```python
from build123d import *

# Parameters (mm, degrees)
BOSS_EXTRUDE1_DEPTH = 11.5
SKETCH2_R           = 1
BOSS_EXTRUDE2_DEPTH = 1.5


with BuildPart() as part:
    # Sketch1 → Boss-Extrude1 (new body)
    with BuildSketch(Plane.XY):
        Polygon((7.5, 5.75), (-7.5, 5.75), (-7.5, -5.75), (-6, -5.75), (-6, 4.25), (6, 4.25), (6, -5.75), (7.5, -5.75), align=None)
    extrude(amount=-BOSS_EXTRUDE1_DEPTH)

    # Sketch2 → Boss-Extrude2 (add)
    with BuildSketch(Plane.XZ.offset(5.75)):
        with BuildLine():
            Line((-7.5, -10.75), (-7.5, -0.75))
            ThreePointArc((-7.5, -0.75), (-12.5, -5.75), (-7.5, -10.75))
        make_face()
        with Locations((-9.5, -4)):
            Circle(SKETCH2_R, mode=Mode.SUBTRACT)
        with BuildLine():
            Line((7.5, -0.75), (7.5, -10.75))
            ThreePointArc((7.5, -10.75), (12.5, -5.75), (7.5, -0.75))
        make_face()
        with Locations((9.5, -4)):
            Circle(SKETCH2_R, mode=Mode.SUBTRACT)
    extrude(amount=-BOSS_EXTRUDE2_DEPTH)


solid = part.part
```
Source: CAD feature listing. Evaluate the final solid. Frame: model axes, mm. A direction names the side the tool comes from. Give positions to 0.01 mm unless a question says otherwise; leave off trailing zeros. Loops run counter-clockwise (first coordinate to the right, second up) from the corner with the lowest first, then second, coordinate; pieces in that order, holes last. Notation, with made-up numbers: (-35, 17) - (-22, 17) arc R25 cw to (-22, 49) - close; hole circle Ø7 at (-3.5, 15). An arc over 180 degrees is marked (long way). Use CSV: the item, a comma, the result in double quotes. Start each with the question number.
1. Section C-C (z = -3.25). Output: boundary loops of the cut face in (x, y).
2. Reachability of faces 1 (the flat face through (9, -4.25, -6)), 2 (the flat face through (0, 5.75, -6)), 3 (the flat face through (6, -1, -6)), 4 (the flat face through (-9, -4.25, -6)) from +Z, -Z, +X, -X, +Y, -Y: full face, straight path, thin tool, end or side. Return the list, or none.
3. Section A-A (y = -2.5). Output: boundary loops of the cut face in (x, z).
4. Draft query along X for faces 5 (the flat face through (0, 4.25, -6)), 6 (the flat face through (8, -5.75, -6)), 7 (the cylindrical face through (8.763, -5.01, -3.324)), 8 (the cylindrical face through (12.5, -5.01, -5.86)). Return one class per face: +X half, -X half, draft (parallel to the pull), parting line (faces both ways), or undercut.
5. Section D-D (x = -9.5). Output: boundary loops of the cut face in (y, z), then the cut area to 3 significant figures.
6. Ray query, L1, parallel to X at y = 2.75, z = -9.5; L2, parallel to Y at x = -9, z = -6.75; L3, parallel to Y at x = 2, z = -7.5. Return the intervals inside material, ascending.
7. Pin query (flat end, axial travel): pin 1 (3 mm diameter, centred on x = -9.5, z = -4, fed in from +Y); pin 2 (1 mm diameter, centred on y = 2.5, z = -2.5, fed in from -X); pin 3 (3 mm diameter, centred on y = 2, z = -4.5, fed in from +X). Return the tip coordinate at first contact, or that it passes through.
8. Section B-B (z = -5.75). Output: boundary loops of the cut face in (x, y).
Response:
1,outline,"(-11.83, -5.75) - (-10.16, -5.75) - (-10.16, -4.25) - (-11.83, -4.25) - close; (-8.84, -5.75) - (-6, -5.75) - (-6, 4.25) - (6, 4.25) - (6, -5.75) - (8.84, -5.75) - (8.84, -4.25) - (7.5, -4.25) - (7.5, 5.75) - (-7.5, 5.75) - (-7.5, -4.25) - (-8.84, -4.25) - close; (10.16, -5.75) - (11.83, -5.75) - (11.83, -4.25) - (10.16, -4.25) - close"
2,face 1,"+Z, -Z, +X, +Y"
2,face 2,"+Z, -Z, +X, -X, +Y"
2,face 3,"+Z, -Z, -Y"
2,face 4,"+Z, -Z, -X, +Y"
3,outline,"(-7.5, -11.5) - (-6, -11.5) - (-6, 0) - (-7.5, 0) - close; (6, -11.5) - (7.5, -11.5) - (7.5, 0) - (6, 0) - close"
4,face 5,"undercut"
4,face 6,"draft"
4,face 7,"undercut"
4,face 8,"+X half"
5,outline,"(-5.75, -10.33) - (-4.25, -10.33) - (-4.25, -5) - (-5.75, -5) - close; (-5.75, -3) - (-4.25, -3) - (-4.25, -1.17) - (-5.75, -1.17) - close"
5,area,"10.7 mm²"
6,L1,"-7.5 to -6, 6 to 7.5"
6,L2,"-5.75 to -4.25"
6,L3,"4.25 to 5.75"
7,pin 1,"y = -4.25"
7,pin 2,"x = -7.5"
7,pin 3,"x = 7.5"
8,outline,"(-12.5, -5.75) - (-6, -5.75) - (-6, 4.25) - (6, 4.25) - (6, -5.75) - (12.5, -5.75) - (12.5, -4.25) - (7.5, -4.25) - (7.5, 5.75) - (-7.5, 5.75) - (-7.5, -4.25) - (-12.5, -4.25) - close"
